Verification items for this drawing (mm, ordinates from the low corner). A direction names the side the tool comes from. Round coordinates to 2 decimals unless told otherwise and drop trailing zeros. Loops run counter-clockwise (first coordinate to the right, second up) from the corner with the lowest first, then second, coordinate; pieces in that order, holes last. Notation, with made-up numbers: (15.25, 2) -> (58.25, 2) arc R22 ccw to (58.25, 13) -> close; hole circle Ø2 at (-14.5, 74). An arc over 180 degrees is marked (long way). Use a Markdown table: item, result. Add a question column.
Q1. Sectioned sample at B-B, the plane z = 1.65. Enter the section's corners in (x, y), then the cut area to 3 significant figures.
Q2. Sectioned sample at D-D, the plane x = 2. Enter the section's corners in (y, z) (3 decimals), then the cut area to 3 significant figures.
Q3. Set-up check for the marked faces 4, 5, 6 and 7: record each of +Z, -Z, +X, -X, +Y, -Y from which the full face is reachable in a straight line by a thin tool's end or side.
Q4. Sectioned sample at A-A, the plane y = 7.75. Enter the section's corners in (x, z) (3 decimals), then the cut area to 3 significant figures.
Q5. Sectioned sample at C-C, the plane x = 13. Enter the section's corners in (y, z) (3 decimals), then the cut area to 3 significant figures.
Q6. Gauge pin test, flat ends, axial feed: P1, Ø1, axis at x = 2.5, z = 1, coming from the -Y side; P2, Ø1.5, axis at y = 3, z = 0.5, coming from the -X side. Record the tip position at first contact, or that the pin passes through.
Q7. Release check for a two-part mould opening along X. For the marked faces 1, 2 and 3 record: released by +X, released by -X, zero draft, split by the parting line, or undercut.
Q8. Material ranges on L1, parallel to X at y = 11, z = 2.7; L2, parallel to X at y = 3, z = 1.15; L3, parallel to Y at x = 27, z = 0.55, recorded low to high.
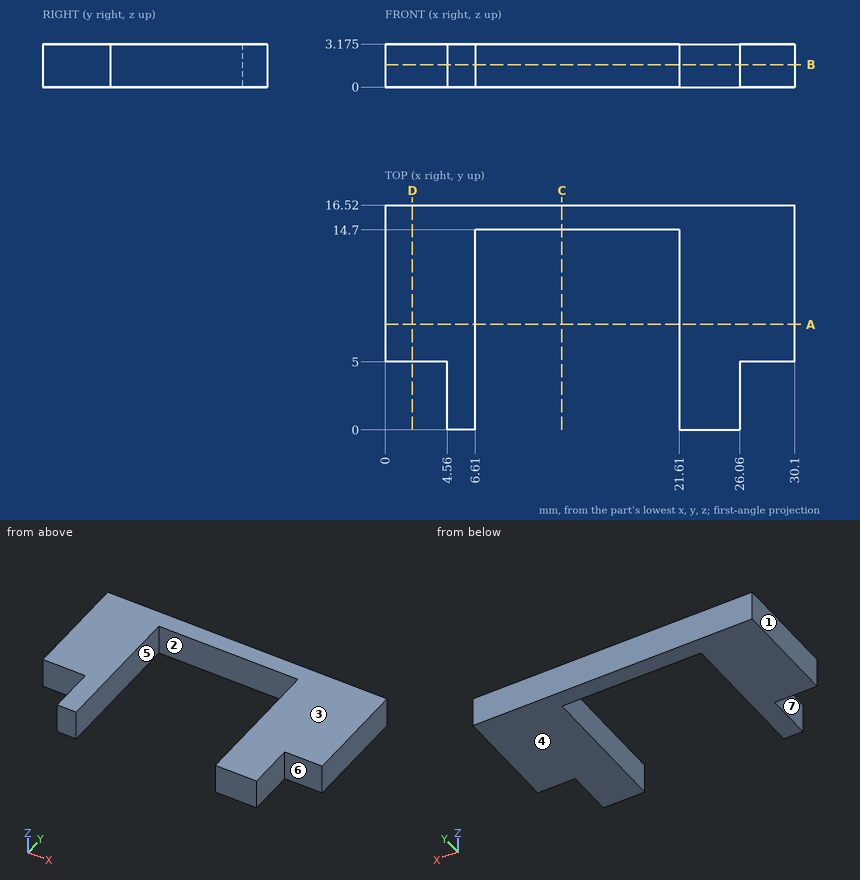
Values:
| question | item | result |
|---|---|---|
| 1 | outline | (0, 5) -> (4.56, 5) -> (4.56, 0) -> (6.61, 0) -> (6.61, 14.7) -> (21.61, 14.7) -> (21.61, 0) -> (26.06, 0) -> (26.06, 5) -> (30.1, 5) -> (30.1, 16.52) -> (0, 16.52) -> close |
| 1 | area | 234 mm^2 |
| 2 | outline | (5, 0) -> (16.52, 0) -> (16.52, 3.175) -> (5, 3.175) -> close |
| 2 | area | 36.6 mm^2 |
| 3 | face 4 | -Z, +X, -X, +Y, -Y |
| 3 | face 5 | +Z, -Z, -Y |
| 3 | face 6 | +Z, -Z, +X, -Y |
| 3 | face 7 | +Z, -Z, -X, -Y |
| 4 | outline | (0, 0) -> (6.61, 0) -> (6.61, 3.175) -> (0, 3.175) -> close; (21.61, 0) -> (30.1, 0) -> (30.1, 3.175) -> (21.61, 3.175) -> close |
| 4 | area | 47.9 mm^2 |
| 5 | outline | (14.7, 0) -> (16.52, 0) -> (16.52, 3.175) -> (14.7, 3.175) -> close |
| 5 | area | 5.78 mm^2 |
| 6 | P1 | y = 5 |
| 6 | P2 | x = 4.56 |
| 7 | face 1 | released by -X |
| 7 | face 2 | undercut |
| 7 | face 3 | zero draft |
| 8 | L1 | 0 to 6.61, 21.61 to 30.1 |
| 8 | L2 | 4.56 to 6.61, 21.61 to 26.06 |
| 8 | L3 | 5 to 16.52 |
